```python
from build123d import *

# Parameters (mm, degrees)
SKETCH1_W           = 66
SKETCH1_H           = 70
BOSS_EXTRUDE1_DEPTH = 2
SKETCH2_W           = 2
SKETCH2_H           = 20
BOSS_EXTRUDE2_DEPTH = 2
SKETCH3_W           = 20
SKETCH3_H           = 2
BOSS_EXTRUDE3_DEPTH = 2
SKETCH8_W           = 5
SKETCH8_H           = 5
CUT_EXTRUDE4_DEPTH  = 10


with BuildPart() as part:
    # Sketch1 → Boss-Extrude1 (new body)
    with BuildSketch(Plane.XY):
        Rectangle(SKETCH1_W, SKETCH1_H)
    extrude(amount=BOSS_EXTRUDE1_DEPTH)

    # Sketch2 → Boss-Extrude2 (add)
    with BuildSketch(Plane(origin=(0, 0, 0), x_dir=(-1, 0, 0), z_dir=(0, 0, -1))):
        with Locations((34, -15)):
            Rectangle(SKETCH2_W, SKETCH2_H)
        with Locations((34, 15)):
            Rectangle(SKETCH2_W, SKETCH2_H)
        with Locations((-34, -15)):
            Rectangle(SKETCH2_W, SKETCH2_H)
        with Locations((-34, 15)):
            Rectangle(SKETCH2_W, SKETCH2_H)
    extrude(amount=-BOSS_EXTRUDE2_DEPTH)

    # Sketch3 → Boss-Extrude3 (add)
    with BuildSketch(Plane(origin=(0, 0, 0), x_dir=(-1, 0, 0), z_dir=(0, 0, -1))):
        with Locations((-15, 36)):
            Rectangle(SKETCH3_W, SKETCH3_H)
        with Locations((15, 36)):
            Rectangle(SKETCH3_W, SKETCH3_H)
        with Locations((-15, -36)):
            Rectangle(SKETCH3_W, SKETCH3_H)
        with Locations((15, -36)):
            Rectangle(SKETCH3_W, SKETCH3_H)
    extrude(amount=-BOSS_EXTRUDE3_DEPTH)

    # Sketch8 → Cut-Extrude4 (cut)
    with BuildSketch(Plane(origin=(0, 0, 0), x_dir=(-1, 0, 0), z_dir=(0, 0, -1))):
        with Locations((-12.5, -12.550886484)):
            Rectangle(SKETCH8_W, SKETCH8_H)
        with Locations((-12.5, -7.550886484)):
            Rectangle(SKETCH8_W, SKETCH8_H)
        with Locations((-7.5, -7.550886484)):
            Rectangle(SKETCH8_W, SKETCH8_H)
        with Locations((-12.5, 2.449113516)):
            Rectangle(SKETCH8_W, SKETCH8_H)
        with Locations((-2.5, 7.449113516)):
            Rectangle(SKETCH8_W, SKETCH8_H)
        with Locations((-2.5, 12.449113516)):
            Rectangle(SKETCH8_W, SKETCH8_H)
        with Locations((2.5, 12.449113516)):
            Rectangle(SKETCH8_W, SKETCH8_H)
        with Locations((7.5, 12.449113516)):
            Rectangle(SKETCH8_W, SKETCH8_H)
        with Locations((12.5, 12.449113516)):
            Rectangle(SKETCH8_W, SKETCH8_H)
        with Locations((12.5, 7.449113516)):
            Rectangle(SKETCH8_W, SKETCH8_H)
        with Locations((12.5, 2.449113516)):
            Rectangle(SKETCH8_W, SKETCH8_H)
        with Locations((12.5, -2.550886484)):
            Rectangle(SKETCH8_W, SKETCH8_H)
        with Locations((7.5, -2.550886484)):
            Rectangle(SKETCH8_W, SKETCH8_H)
        with Locations((7.5, -7.550886484)):
            Rectangle(SKETCH8_W, SKETCH8_H)
        with Locations((7.5, -12.550886484)):
            Rectangle(SKETCH8_W, SKETCH8_H)
    extrude(amount=-CUT_EXTRUDE4_DEPTH, mode=Mode.SUBTRACT)


solid = part.part
```
Here's how the part is built. I have some questions about the finished solid (model axes, mm). A direction names the side the tool comes from. Give positions to 0.01 mm unless a question says otherwise; leave off trailing zeros. Loops run counter-clockwise (first coordinate to the right, second up) from the corner with the lowest first, then second, coordinate; pieces in that order, holes last. Notation, with made-up numbers: M -11,33.25 L 31,33.25 A27 cw 31,63.25 Z; hole C 61,36 d2. An arc over 180 degrees is marked long. Put each result on its own line as item: value. Start each with the question number.
(1) Will these pins go through, and if not, where does the flat tip stop? pin 1 Ø1 at (y, z) = (-36, 1) entering from +X; pin 2 Ø1 at (y, z) = (36, 1) entering from -X.
(2) For faces 4 (the flat face through (5, -8, 1)), 5 (the flat face through (0, 35, 1)), 6 (the flat face through (34, 25, 1)), which set-ups out of +Z, -Z, +X, -X, +Y, -Y let a thin tool reach every point of the face, with its end or its side?
(3) I want a section at B-B on x = 7. Please give me the cut outline in (y, z).
(4) If we mould it in two halves opening along X, with no side actions, what happens to faces 1 (the flat face through (10, -13, 1)), 2 (the flat face through (34, -25, 1)), 3 (the flat face through (-33, 0, 1))? For each: +X half, -X half, draft (parallel to the pull), parting line (faces both ways), or undercut.
(5) I want a section at A-A on y = 11.5. Please give me the cut outline in (x, z), then the cut area to 3 significant figures.
(6) I want a section at D-D on x = -28. Please give me the cut outline in (y, z), then the cut area to 3 significant figures.
(7) I want a section at C-C on y = 2. Please give me the cut outline in (x, z), then the cut area to 3 significant figures.
(8) I need wall thicknesses on line 1 along X through (y, z) = (-9, 1.8); line 2 along X through (y, z) = (-14, 0.45); line 3 along Y through (x, z) = (10.5, 0.6). Which ranges of each line are inside material? Lowest first, please. Write a range as [from, to].
Answer block:
1. pin 1: x = 25
1. pin 2: x = -25
2. face 4: +Z, -Z
2. face 5: +Z, -Z, +Y
2. face 6: +Z, -Z, +X, +Y
3. outline: M -37,0 L -10.05,0 L -10.05,2 L -37,2 Z; M -5.05,0 L 37,0 L 37,2 L -5.05,2 Z
4. face 1: undercut
4. face 2: draft
4. face 3: -X half
5. outline: M -35,0 L -15,0 L -15,2 L -35,2 Z; M 5,0 L 35,0 L 35,2 L 5,2 Z
5. area: 100 mm^2
6. outline: M -35,0 L 35,0 L 35,2 L -35,2 Z
6. area: 140 mm^2
7. outline: M -33,0 L -15,0 L -15,2 L -33,2 Z; M -10,0 L 10,0 L 10,2 L -10,2 Z; M 15,0 L 33,0 L 33,2 L 15,2 Z
7. area: 112 mm^2
8. line 1: [-35, -10], [-5, 5], [15, 35]
8. line 2: [-35, -10], [-5, 10], [15, 35]
8. line 3: [-37, -15.05], [-5.05, -0.05], [4.95, 37]
